Geometry check sheet. Reference: the model listing, model coordinates, mm. A direction names the side the tool comes from. Round coordinates to 2 decimals unless told otherwise and drop trailing zeros. Loops run counter-clockwise (first coordinate to the right, second up) from the corner with the lowest first, then second, coordinate; pieces in that order, holes last. Notation, with made-up numbers: M 23,78 L 65,78 A21 ccw 65,94 Z; hole C 43.5,12.5 d11. An arc over 180 degrees is marked long. Use one line per item in the form item = value. Start each with the question number.
1. Cross-section at D-D (x = -61). Record the boundary of the cut face in (y, z).
2. Material ranges on line 1 (Z direction, x = -92, y = -164); line 2 (X direction, y = -87, z = 21); line 3 (Z direction, x = -57, y = -91), recorded low to high.
3. Go/stop test with flat-tipped pins: pin 1 (5 mm diameter, centred on y = -95, z = 40.5, fed in from -X); pin 2 (7 mm diameter, centred on x = -104, y = -147.5, fed in from +Z); pin 3 (2 mm diameter, centred on x = -56, z = 8.5, fed in from +Y). Record where each tip stops, or that it passes through.
4. Cross-section at C-C (y = -145.5). Record the boundary of the cut face in (x, z), then the cut area to 3 significant figures.
5. Draft check along X on faces 1 (the flat face through (-97, -156, 15)), 2 (the flat face through (-113.324, -77.427, 14.79)), 3 (the cylindrical face through (-51.04, -108.35, 2.46)). Enter one of: pulls with the +X half, pulls with the -X half, needs draft (parallel to the pull), parting line crosses it, or undercut.
6. Set-up check for faces 4 (the flat face through (-89.254, -92.404, 14.79)), 5 (the flat face through (-98.314, -156.642, 9.93)), 6 (the cylindrical face through (-104.42, -150.95, 2.46)): record each of +Z, -Z, +X, -X, +Y, -Y from which the full face is reachable in a straight line by a thin tool's end or side.
7. Cross-section at A-A (z = 50.5). Record the boundary of the cut face in (x, y).
8. Cross-section at B-B (x = -91.5). Record the boundary of the cut face in (y, z), then the cut area to 3 significant figures.
```python
from build123d import *

# Parameters (mm, degrees)
ESTRUSIONE_ESTRUSIONE1_DEPTH = 5
ESTRUSIONE_ESTRUSIONE2_DEPTH = 7
ESTRUSIONE_ESTRUSIONE3_DEPTH = 3
ESTRUSIONE_ESTRUSIONE4_DEPTH = 52
TAGLIO_ESTRUSIONE2_DEPTH     = 27
ESTRUSIONE_ESTRUSIONE8_DEPTH = 10
ESTRUSIONE_ESTRUSIONE6_DEPTH = 30
SCHIZZO10_W                  = 14
SCHIZZO10_H                  = 7
ESTRUSIONE_ESTRUSIONE7_DEPTH = 0.3


with BuildPart() as part:
    # Schizzo1 → Estrusione-Estrusione1 (new body)
    with BuildSketch(Plane.XY):
        with BuildLine():
            Line((-82.995904107, -166.584374689), (-92.877799089, -168.116742646))
            ThreePointArc((-92.877799089, -168.116742646), (-110.220012955, -164.040092202), (-119.840608042, -149.046239769))
            ThreePointArc((-119.840608042, -149.046239769), (-118.364815633, -130.917411526), (-107.867932944, -116.063192243))
            Line((-107.867932944, -116.063192243), (-84.49215827, -97.259651129))
            ThreePointArc((-84.49215827, -97.259651129), (-67.733683115, -90.189581316), (-49.709718148, -92.632748029))
            ThreePointArc((-49.709718148, -92.632748029), (-37.125664022, -105.242785395), (-36.859828578, -123.055724291))
            Line((-36.859828578, -123.055724291), (-40.474113425, -132.379722631))
            Line((-40.474113425, -132.379722631), (-54.467826156, -126.955304689))
            Line((-54.467826156, -126.955304689), (-50.853541308, -117.631306349))
            ThreePointArc((-50.853541308, -117.631306349), (-51.095893898, -108.22813541), (-57.953355129, -101.789689638))
            ThreePointArc((-57.953355129, -101.789689638), (-68.520842721, -100.735914417), (-78.224311232, -105.051576021))
            Line((-78.224311232, -105.051576021), (-101.600085906, -123.855117134))
            ThreePointArc((-101.600085906, -123.855117134), (-107.894780127, -132.408424149), (-109.129903142, -142.956253658))
            ThreePointArc((-109.129903142, -142.956253658), (-104.310440062, -151.034071069), (-95.177618995, -153.285723315))
            Line((-95.177618995, -153.285723315), (-85.295724012, -151.753355358))
            Line((-85.295724012, -151.753355358), (-82.995904107, -166.584374689))
        make_face()
    extrude(amount=ESTRUSIONE_ESTRUSIONE1_DEPTH)

    # Schizzo2 → Estrusione-Estrusione2 (add)
    with BuildSketch(Plane.XY.offset(5)):
        with BuildLine():
            Line((-36.859828578, -123.055724291), (-50.830842779, -117.640105037))
            ThreePointArc((-50.830842779, -117.640105037), (-50.298673229, -115.886666013), (-50.034997321, -114.073318872))
            Line((-50.034997321, -114.073318872), (-35.811832194, -119.586680021))
            ThreePointArc((-35.811832194, -119.586680021), (-36.269524014, -121.341233275), (-36.859828578, -123.055724291))
        make_face()
        with BuildLine():
            Line((-96.490830562, -168.397042736), (-98.828360202, -153.322841843))
            ThreePointArc((-98.828360202, -153.322841843), (-97.000632762, -153.453858051), (-95.173888567, -153.309779998))
            Line((-95.173888567, -153.309779998), (-92.877799089, -168.116742646))
            ThreePointArc((-92.877799089, -168.116742646), (-94.678957246, -168.325951195), (-96.490830562, -168.397042736))
        make_face()
    extrude(amount=ESTRUSIONE_ESTRUSIONE2_DEPTH)

    # Schizzo3 → Estrusione-Estrusione3 (add)
    with BuildSketch(Plane.XY.offset(12)):
        with BuildLine():
            Line((-42.270578454, -137.014176653), (-36.859828578, -123.055724291))
            ThreePointArc((-36.859828578, -123.055724291), (-36.269524014, -121.341233275), (-35.811832194, -119.586680021))
            Line((-35.811832194, -119.586680021), (-50.034997321, -114.073318872))
            ThreePointArc((-50.034997321, -114.073318872), (-50.288758238, -115.888878313), (-50.830842779, -117.640105037))
            Line((-50.830842779, -117.640105037), (-53.115040991, -123.532795079))
            Line((-53.115040991, -123.532795079), (-42.270578454, -137.014176653))
        make_face()
        with BuildLine():
            Line((-96.490830562, -168.397042736), (-98.828360202, -153.322841843))
            ThreePointArc((-98.828360202, -153.322841843), (-97.000596453, -153.464016791), (-95.173888567, -153.309779998))
            Line((-95.173888567, -153.309779998), (-88.928612449, -152.34133609))
            Line((-88.928612449, -152.34133609), (-78.084149913, -165.822717664))
            Line((-78.084149913, -165.822717664), (-92.877799089, -168.116742646))
            ThreePointArc((-92.877799089, -168.116742646), (-94.678957246, -168.325951195), (-96.490830562, -168.397042736))
        make_face()
    extrude(amount=ESTRUSIONE_ESTRUSIONE3_DEPTH)

    # Schizzo4 → Estrusione-Estrusione4 (add)
    with BuildSketch(Plane.XY.offset(5)):
        Polygon((-101.600085906, -123.855117134), (-78.224311232, -105.051576021), (-84.49215827, -97.259651129), (-107.867932944, -116.063192243), align=None)
    extrude(amount=ESTRUSIONE_ESTRUSIONE4_DEPTH)

    # Schizzo5 → Taglio-Estrusione2 (cut)
    with BuildSketch(Plane.XY.offset(57)):
        Polygon((-97.246900104, -116.503262037), (-97.873684808, -115.724069548), (-98.141552252, -109.009291291), (-98.517623074, -108.541775798), (-93.842468139, -104.781067575), (-93.466397317, -105.248583068), (-86.96498996, -106.949083694), (-86.338205256, -107.728276184), align=None)
    extrude(amount=-TAGLIO_ESTRUSIONE2_DEPTH, mode=Mode.SUBTRACT)

    # Schizzo6 → Estrusione-Estrusione8 (add)
    with BuildSketch(Plane.XY.offset(5)):
        Polygon((-97.823256998, -159.87152255), (-97.519846298, -161.848374074), (-97.50663255, -161.846365055), (-97.813109395, -159.869965078), align=None)
        with BuildLine():
            Line((-104.107224721, -120.738347178), (-105.360794128, -119.1799622))
            ThreePointArc((-105.360794128, -119.1799622), (-115.28727508, -135.493487076), (-112.492970749, -154.384172115))
            ThreePointArc((-112.492970749, -154.384172115), (-106.191101066, -160.49275607), (-97.519846298, -161.848374074))
            Line((-97.519846298, -161.848374074), (-97.823256998, -159.87152255))
            ThreePointArc((-97.823256998, -159.87152255), (-105.298812913, -158.702833766), (-110.731703589, -153.436576214))
            ThreePointArc((-110.731703589, -153.436576214), (-113.327097811, -135.89060806), (-104.107224721, -120.738347178))
        make_face()
        with BuildLine():
            ThreePointArc((-43.853805634, -116.458338954), (-43.393471858, -108.905997429), (-47.373234104, -102.470839142))
            ThreePointArc((-47.373234104, -102.470839142), (-63.955496248, -96.175948212), (-80.731450047, -101.934806064))
            Line((-80.731450047, -101.934806064), (-81.985019455, -100.376421086))
            ThreePointArc((-81.985019455, -100.376421086), (-63.923362402, -94.176206375), (-46.070241465, -100.953535552))
            ThreePointArc((-46.070241465, -100.953535552), (-41.453924934, -108.417983362), (-41.987888093, -117.178305432))
            Line((-41.987888093, -117.178305432), (-43.853805634, -116.458338954))
        make_face()
        Polygon((-43.857501376, -116.467917109), (-43.853805634, -116.458338954), (-41.987888093, -117.178305432), (-41.99269947, -117.190774947), align=None)
    extrude(amount=ESTRUSIONE_ESTRUSIONE8_DEPTH)

    # Schizzo9 → Estrusione-Estrusione6 (add)
    with BuildSketch(Plane(origin=(0, 0, 0), x_dir=(-1, 0, 0), z_dir=(0, 0, -1))):
        with BuildLine():
            Line((93.885019226, -87.68303048), (84.49215827, -97.259651129))
            Line((84.49215827, -97.259651129), (107.867932944, -116.063192243))
            Line((107.867932944, -116.063192243), (115.209386763, -104.836413728))
            ThreePointArc((115.209386763, -104.836413728), (117.333034353, -99.111871829), (116.768742523, -93.032247353))
            Line((116.768742523, -93.032247353), (123.036589561, -85.240322461))
            Line((123.036589561, -85.240322461), (119.140627115, -82.106398942))
            Line((119.140627115, -82.106398942), (111.879963827, -91.132551409))
            ThreePointArc((111.879963827, -91.132551409), (97.276918838, -105.29783483), (107.984001382, -87.99862789))
            Line((107.984001382, -87.99862789), (115.24466467, -78.972475424))
            Line((115.24466467, -78.972475424), (111.348702224, -75.838551905))
            Line((111.348702224, -75.838551905), (105.080855186, -83.630476796))
            ThreePointArc((105.080855186, -83.630476796), (99.021531527, -84.382045715), (93.885019226, -87.68303048))
        make_face()
    extrude(amount=-ESTRUSIONE_ESTRUSIONE6_DEPTH)

    # Schizzo10 → Estrusione-Estrusione7 (add)
    with BuildSketch(Plane(origin=(18.694228144, -23.239881369, 0), x_dir=(0.779192489117125, 0.6267847037886766, 0), z_dir=(-0.6267847037886766, 0.779192489117125, 0))):
        with Locations((-141.796516737, -33.5)):
            Rectangle(SCHIZZO10_W, SCHIZZO10_H)
    extrude(amount=ESTRUSIONE_ESTRUSIONE7_DEPTH)


solid = part.part
```
Reported:
q1.outline = M -100.91,0 L -89.96,0 L -89.96,5 L -94.38,5 L -94.38,15 L -96.39,15 L -96.39,5 L -100.91,5 Z
q2.line_1 = 0 to 5, 12 to 15
q2.line_2 = -121.62 to -115.2, -108.79 to -94.61
q2.line_3 = 0 to 5
q3.pin_1 = -84.79
q3.pin_2 = 5
q3.pin_3 = -95.16
q4.outline = M -120.32,0 L -108.48,0 L -108.48,5 L -113.47,5 L -113.47,15 L -115.5,15 L -115.5,5 L -120.32,5 Z
q4.area = 79.5 mm²
q5.face_1 = needs draft
q5.face_2 = pulls with the -X half
q5.face_3 = undercut
q6.face_4 = +Z, -Z, +Y
q6.face_5 = +Z
q6.face_6 = +Z, -Z
q7.outline = M -107.87,-116.06 L -101.6,-123.86 L -78.22,-105.05 L -84.49,-97.26 L -93.84,-104.78 L -93.47,-105.25 L -86.96,-106.95 L -86.34,-107.73 L -97.25,-116.5 L -97.87,-115.72 L -98.14,-109.01 L -98.52,-108.54 Z
q8.outline = M -167.9,0 L -152.72,0 L -152.72,5 L -167.9,5 Z; M -167.9,12 L -152.74,12 L -152.74,15 L -167.9,15 Z; M -115.73,0 L -90.11,0 L -90.11,30 L -102.9,30 L -102.9,57 L -105.76,57 L -105.76,30 L -111.5,30 L -111.5,37 L -111.88,37 L -111.88,57 L -115.73,57 Z
q8.area = 1,070 mm²
